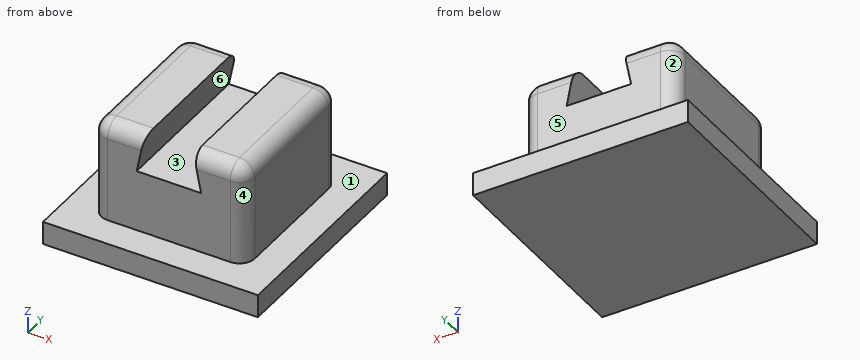
```python
from build123d import *

# Parameters (mm, degrees)
F0_W     = 14
F0_H     = 14
F0_W_2   = 10
F0_H_2   = 10
F1_DEPTH = 1.5
F2_DEPTH = 8
F4_DEPTH = 25
F5_R     = 1


with BuildPart() as f1:
    # F0 (on Top) → F1 (new body)
    with BuildSketch(Plane.XY):
        Rectangle(F0_W, F0_H)
        Rectangle(F0_W_2, F0_H_2, mode=Mode.SUBTRACT)
    extrude(amount=F1_DEPTH)

    # F0 (on Top) → F2 (join)
    with BuildSketch(Plane.XY):
        Rectangle(F0_W_2, F0_H_2)
    extrude(amount=F2_DEPTH)

    # F3 (on face) → F4 (cut)
    with BuildSketch(Plane.XZ.offset(5)):
        Polygon((1.6, 8), (-1.6, 8), (-2.1, 5.5), (2.1, 5.5), align=None)
    extrude(amount=-F4_DEPTH, mode=Mode.SUBTRACT)

    # F5
    f5_edges = [f1.edges().sort_by_distance(p)[0] for p in [
        (-5, 0, 8),
        (3.3, -5, 8),
        (-3.3, -5, 8),
        (-3.3, 5, 8),
        (3.3, 5, 8),
        (-5, 5, 4.75),
        (-5, -5, 4.75),
        (5, -5, 4.75),
        (5, 5, 4.75),
        (5, 0, 8),
    ]]
    fillet(f5_edges, radius=F5_R)


solid = f1.part
```
CAD build for the part. Positions are in the model's coordinates, mm. Face numbers are marked on the shaded views. A direction names the side the tool comes from. Round coordinates to 2 decimals unless told otherwise and drop trailing zeros. Write each loop counter-clockwise with the first axis right and the second up, starting at its lowest first coordinate (ties: lowest second). Pieces come first, ordered by that corner, then holes.
Item 1: Band-saw the part on D-D on y = -4.25. Write the cut outline in (x, z).
Filled in:
outline: (-7, 0) - (7, 0) - (7, 1.5) - (4.97, 1.5) - (4.97, 7) arc R0.97 ccw to (4, 7.97) - (1.61, 7.97) - (2.1, 5.5) - (-2.1, 5.5) - (-1.61, 7.97) - (-4, 7.97) arc R0.97 ccw to (-4.97, 7) - (-4.97, 1.5) - (-7, 1.5) - close
Item 2: Band-saw the part on A-A on z = 6.75. Write the cut outline in (x, y).
Filled in:
outline: (-5, -4) arc R1 ccw to (-4, -5) - (-1.85, -5) - (-1.85, 5) - (-4, 5) arc R1 ccw to (-5, 4) - close; (1.85, -5) - (4, -5) arc R1 ccw to (5, -4) - (5, 4) arc R1 ccw to (4, 5) - (1.85, 5) - close
Item 3: Drop flat-ended pins along their axis: pin 1 Ø1 at (y, z) = (-3, 5.5) entering from -X; pin 2 Ø3 at (x, z) = (0, 5) entering from +Y; pin 3 Ø4 at (x, y) = (5, -4.5) entering from +Z; pin 4 Ø1.6 at (y, z) = (1.5, 5.5) entering from +X. Give the stop position or say it passes through.
Filled in:
pin 1: stops at x = -5
pin 2: stops at y = 5
pin 3: stops at z = 8
pin 4: stops at x = 5
Item 4: Band-saw the part on B-B on z = 3.25. Write the cut outline in (x, y), then the cut area to 3 significant figures.
Filled in:
outline: (-5, -4) arc R1 ccw to (-4, -5) - (4, -5) arc R1 ccw to (5, -4) - (5, 4) arc R1 ccw to (4, 5) - (-4, 5) arc R1 ccw to (-5, 4) - close
area: 99.1 mm2
Item 5: Mould opens along X. For the marked faces 4, 5 and 6 say: released by +X, released by -X, zero draft, split by the parting line, or undercut.
Filled in:
face 4: released by +X
face 5: zero draft
face 6: undercut
Item 6: Band-saw the part on C-C on x = -1. Write the cut outline in (y, z), then the cut area to 3 significant figures.
Filled in:
outline: (-7, 0) - (7, 0) - (7, 1.5) - (5, 1.5) - (5, 5.5) - (-5, 5.5) - (-5, 1.5) - (-7, 1.5) - close
area: 61.0 mm2
Item 7: Tool access for the marked faces 1, 2 and 3: list every direction of +Z, -Z, +X, -X, +Y, -Y with a clear straight run to the whole face (end or side of a thin tool).
Filled in:
face 1: +Z
face 2: +Z, -X, +Y
face 3: +Y, -Y
Item 8: Drill centre lines: L1, parallel to Y at x = 2, z = 2.25; L2, parallel to Z at x = -2.25, y = -5.75; L3, parallel to Z at x = 1.25, y = -0.75. Where is each one in solid material? Low to high.
Filled in:
L1: y = -5 to 5
L2: z = 0 to 1.5
L3: z = 0 to 5.5
